from build123d import *

# Parameters (mm, degrees)
SKETCH_1_W          = 8
SKETCH_1_H          = 21.1
EXTRUDE_1_DEPTH     = 13.55
SKETCH_2_R          = 1.5
SKETCH_2_W          = 0.25
SKETCH_2_H          = 1.5
EXTRUDE_2_DEPTH     = 3.6
CUT_EXTRUDE_1_DEPTH = 12
SKETCH_4_W          = 3.1
SKETCH_4_H          = 1.8
CUT_EXTRUDE_2_DEPTH = 0.01
SKETCH_5_R          = 0.3
EXTRUDE_3_DEPTH     = 3.6


with BuildPart() as part:
    # Эскиз1 → Бобышка-Вытянуть1 (new body)
    with BuildSketch(Plane.XY):
        with Locations((-4, 10.55)):
            Rectangle(SKETCH_1_W, SKETCH_1_H)
    extrude(amount=EXTRUDE_1_DEPTH)

    # Эскиз2 → Бобышка-Вытянуть2 (add)
    with BuildSketch(Plane(origin=(0, 0, 0), x_dir=(-1, 0, 0), z_dir=(0, 0, -1))):
        with Locations((5.715, 10.8)):
            Circle(SKETCH_2_R)
        with Locations((7.875, 13.85)):
            Rectangle(SKETCH_2_W, SKETCH_2_H)
    extrude(amount=EXTRUDE_2_DEPTH)

    # Эскиз3 → Вырез-Вытянуть1 (cut)
    with BuildSketch(Plane.XZ):
        Polygon((0, 1), (-2, 1), (-2, 2.3), (-3.2, 2.3), (-3.2, 4), (-6, 4), (-6, 11.05), (0, 11.05), align=None)
    extrude(amount=-CUT_EXTRUDE_1_DEPTH, mode=Mode.SUBTRACT)

    # Эскиз4 → Вырез-Вытянуть2 (cut)
    with BuildSketch(Plane.XZ):
        with Locations((-5.45, 1.9)):
            Rectangle(SKETCH_4_W, SKETCH_4_H)
    extrude(amount=-CUT_EXTRUDE_2_DEPTH, mode=Mode.SUBTRACT)

    # Зеркальное отражение1: part across plane


with BuildPart() as part_1:
    add(part.part)
    add(part.part.mirror(Plane(origin=(0, 0, 13.55), x_dir=(0, 0, 1), z_dir=(-1, 0, 0))))

    # Эскиз5 → Бобышка-Вытянуть3 (add)
    with BuildSketch(Plane(origin=(0, 0, 0), x_dir=(-1, 0, 0), z_dir=(0, 0, -1))):
        with Locations((-6.325, 7.42)):
            Circle(SKETCH_5_R)
        with Locations((-3.785, 5.9)):
            Circle(SKETCH_5_R)
        with Locations((3.785, 7.42)):
            Circle(SKETCH_5_R)
        with Locations((6.325, 5.9)):
            Circle(SKETCH_5_R)
        with Locations((-4.445, 19.69)):
            Circle(SKETCH_5_R)
        with Locations((-1.905, 19.69)):
            Circle(SKETCH_5_R)
        with Locations((0.635, 19.69)):
            Circle(SKETCH_5_R)
        with Locations((3.175, 19.69)):
            Circle(SKETCH_5_R)
        with Locations((-3.175, 17.15)):
            Circle(SKETCH_5_R)
        with Locations((-0.635, 17.15)):
            Circle(SKETCH_5_R)
        with Locations((1.905, 17.15)):
            Circle(SKETCH_5_R)
        with Locations((4.445, 17.15)):
            Circle(SKETCH_5_R)
    extrude(amount=EXTRUDE_3_DEPTH)


solid = part_1.part
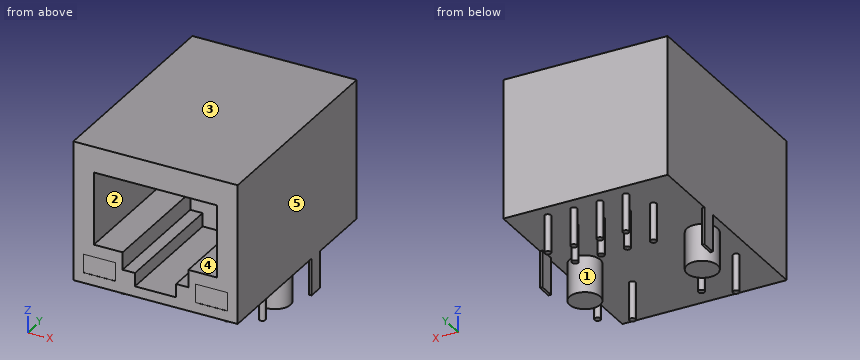
Build history of the part. All positions in model axes, mm. Face numbers are marked on the shaded views. A direction names the side the tool comes from. Round coordinates to 2 decimals unless told otherwise and drop trailing zeros. Write each loop counter-clockwise with the first axis right and the second up, starting at its lowest first coordinate (ties: lowest second). Pieces come first, ordered by that corner, then holes. Notation, with made-up numbers: M 85,11 L 130,11 A22 cw 130,41 Z; hole C 78,31 d6. An arc over 180 degrees is marked long. Answer as a JSON object with one key per item and string values. Group by question number.
(1) Cut at C-C (x = -2.5). Give the cut face in (y, z).
(2) Drill centre lines: L1, parallel to Z at x = -3, y = 8.75; L2, parallel to X at y = 2.5, z = 8.5; L3, parallel to Z at x = -0.75, y = 1.25. Where is each one in solid material? Low to high.
(3) Flat gauge pin, fed straight in: pin 1 (1 mm diameter, centred on x = 3.5, z = 5.5, fed in from -Y). Where does the tip first touch, or does it go through?
(4) Cut at D-D (y = 19.69). Give the cut face in (x, z) (3 decimals), and give its area (3 significant figures).
(5) Cut at A-A (y = 9). Give the cut face in (x, z).
(6) Which spindle directions (+Z, -Z, +X, -X, +Y, -Y) get a long thin tool onto all of the face, cutting with end or side? Do the marked faces 1 and 2. Say none if no direction does.
(7) Mould opens along X. For the marked faces 3, 4 and 5 say: pulls with the +X half, pulls with the -X half, needs draft (parallel to the pull), parting line crosses it, or undercut.
Responses:
{
 "1": {"outline": "M 0,0 L 21.1,0 L 21.1,13.55 L 0,13.55 L 0,11.05 L 12,11.05 L 12,2.3 L 0,2.3 Z"},
 "2": {"L1": "z = 0 to 2.3, 11.05 to 13.55", "L2": "x = -8 to -6, 6 to 8", "L3": "z = 0 to 1, 11.05 to 13.55"},
 "3": {"pin 1": "stops at y = 12"},
 "4": {"outline": "M -8,0 L -3.475,0 L -3.475,-3.6 L -2.875,-3.6 L -2.875,0 L -0.935,0 L -0.935,-3.6 L -0.335,-3.6 L -0.335,0 L 1.605,0 L 1.605,-3.6 L 2.205,-3.6 L 2.205,0 L 4.145,0 L 4.145,-3.6 L 4.745,-3.6 L 4.745,0 L 8,0 L 8,13.55 L -8,13.55 Z", "area": "225 mm2"},
 "5": {"outline": "M -8,0 L 8,0 L 8,13.55 L -8,13.55 Z; hole M -6,4 L -3.2,4 L -3.2,2.3 L -2,2.3 L -2,1 L 2,1 L 2,2.3 L 3.2,2.3 L 3.2,4 L 6,4 L 6,11.05 L -6,11.05 Z"},
 "6": {"face 1": "-Z", "face 2": "-Y"},
 "7": {"face 3": "needs draft", "face 4": "undercut", "face 5": "pulls with the +X half"}
}
